Check sheet for the modelled part. Datum: model origin and axes. Units: mm. Face numbers are marked on the shaded views. A direction names the side the tool comes from. Round coordinates to 2 decimals unless told otherwise and drop trailing zeros. Order: outer loops, then holes, each group sorted by start corner. A loop starts at its lowest first (then second) coordinate and runs counter-clockwise, first axis right, second up.
Q1. Cross-section at A-A on z = 4. Record the cut outline in (x, y) (3 decimals), then the cut area to 4 significant figures.
Q2. Scan lines: probe 1 along X at (y, z) = (-0.5, 7); probe 2 along Y at (x, z) = (-26, 11.5); probe 3 along Y at (x, z) = (10.5, 3.5). Record each from-to range of solid material in increasing order.
Q3. Depth check by flat-ended pin: P1, Ø2, axis at y = -5.5, z = 6.5, coming from the +X side; P2, Ø13, axis at x = 0.5, z = 4, coming from the -Y side; P3, Ø2, axis at x = 34, z = 4.5, coming from the -Y side; P4, Ø10, axis at x = 38.5, y = -15, coming from the +Z side. Enter the tip coordinate at first touch or a pass-through.
Q4. Cross-section at C-C on z = 27. Record the cut outline in (x, y).
Q5. Set-up check for the marked faces 5 and 6: record each of +Z, -Z, +X, -X, +Y, -Y from which the full face is reachable in a straight line by a thin tool's end or side.
Q6. Mould release check, pull along X, two halves, no side actions. Record for the marked faces 1, 2, 3 and 4: +X half, -X half, draft (parallel to the pull), parting line (faces both ways), or undercut.
Q7. Cross-section at B-B on x = -20. Record the cut outline in (y, z).
Q8. Cross-section at D-D on y = -28.5. Record the cut outline in (x, z), then the cut area to 3 significant figures.
Autodesk Inventor part; units mm, degrees
ref_plane "YZ Plane" through (0, 0, 0) normal (1, 0, 0) x (0, 1, 0)
ref_plane "XZ Plane" through (0, 0, 0) normal (0, 1, 0) x (-1, 0, 0)
ref_plane "XY Plane" through (0, 0, 0) normal (0, 0, 1) x (1, 0, 0)
sketch "Sketch2" plane through (0, 0, 0) normal (0, 0, 1) x (1, 0, 0)
  line L0 (-32.475, -3.1) -> (-25.525, -3.1)
  line L1 (-25.525, -3.1) -> (-25.525, -7)
  line L2 (-25.525, -7) -> (-32.475, -7)
  line L3 (-32.475, -7) -> (-32.475, -3.1)
  line L4 (-31.2, 0) -> (-26.8, 0)
  line L5 (-26.8, 0) -> (-26.8, -3.1)
  line L6 (-26.8, -3.1) -> (-31.2, -3.1)
  line L7 (-31.2, -3.1) -> (-31.2, 0)
  line L8 (-35.5, 0) -> (0, 0)
  line L9 (0, 5) -> (-35.5, 5)
  line L10 (-35.5, 5) -> (-35.5, 0)
  line L11 (-29, 6.5254) -> (-29, -10.3092) construction
  line L12 (0, -40.9051) -> (0, 14.4305) construction
  line L13 (32.475, -3.1) -> (25.525, -3.1)
  line L14 (25.525, -3.1) -> (25.525, -7)
  line L15 (25.525, -7) -> (32.475, -7)
  line L16 (32.475, -7) -> (32.475, -3.1)
  line L17 (31.2, 0) -> (26.8, 0)
  line L18 (26.8, 0) -> (26.8, -3.1)
  line L19 (26.8, -3.1) -> (31.2, -3.1)
  line L20 (31.2, -3.1) -> (31.2, 0)
  line L21 (35.5, 0) -> (0, 0)
  line L22 (0, 5) -> (35.5, 5)
  line L23 (35.5, 5) -> (35.5, 0)
  line L24 (29, 6.5254) -> (29, -10.3092) construction
  line L25 (-85.0097, 0) -> (105.1151, 0) construction
  line L26 (35.5, 5) -> (77.9544, -30.0249)
  line L27 (77.9544, -30.0249) -> (75.5, -33)
  line L28 (75.5, -33) -> (35.5, 0)
  line L29 (-35.5, 5) -> (35.5, 5)
  line L30 (35.5, 5) -> (35.5, -7)
  line L31 (35.5, -7) -> (-35.5, -7)
  line L32 (-35.5, -7) -> (-35.5, 5)
  line L33 (-35.5, 5) -> (-57.849, -10.6443)
  line L34 (-57.849, -10.6443) -> (-55.5, -14)
  line L35 (-55.5, -14) -> (-35.5, 0)
  line L36 (-49.6567, -4.9097) -> (-47.3077, -8.2654)
  line L37 (-21.525, -7) -> (-21.525, -4)
  line L38 (-21.525, -4) -> (0, -4)
  line L39 (21.525, -7) -> (21.525, -4)
  line L40 (21.525, -4) -> (0, -4)
  line L41 (-35.5, -7) -> (-45.5, -7)
  line L42 (35.5, -7) -> (43.9848, -7)
  point P0 (-13.25, 5)
  point P1 (-18.25, 5)
  point P2 (29, -7)
  dimension "d1" = 4.4
  dimension "d2" = 6.95
  dimension "d3" = 3.9
  dimension "d4" = 5
  dimension "d5" = 58
  dimension "d6" = 7
  dimension "d7" = 13
  dimension "d28" = 38
  dimension "d29" = 40
  dimension "d30" = 20
  dimension "d31" = 19
  dimension "d32" = 10
  dimension "d37" = 4
  dimension "d38" = 3
extrude "Extrusion1" add sketch "Sketch2" along normal blind 12 contours L0 L1 L2 L3 | L7 L4 L5 L0 | L8 L10 L9 L22 L23 L21 L17 L4 | L35 L36 L33 L10 | L17 L20 L13 L18 | L14 L13 L16 L15 | L26 L27 L28 L23
extrude "Extrusion2" add sketch "Sketch2" along normal blind 40 contours L35 L34 L33 L36
extrude "Extrusion3" add sketch "Sketch2" against normal blind 3 contours L3 L31 L32 L8 L7 L0 | L0 L1 L2 L3 | L7 L4 L5 L0 | L5 L8 L21 L18 L13 L14 L31 L39 L40 L38 L37 L1 L0 | L8 L10 L9 L22 L23 L21 L17 L4 | L41 L35 L32 | L35 L36 L33 L10 | L35 L34 L33 L36 | L17 L20 L13 L18 | L14 L13 L16 L15 | L21 L30 L31 L16 L13 L20 | L26 L27 L28 L23 | L28 L42 L30
properties part number "UnitreeGO2_railmount"
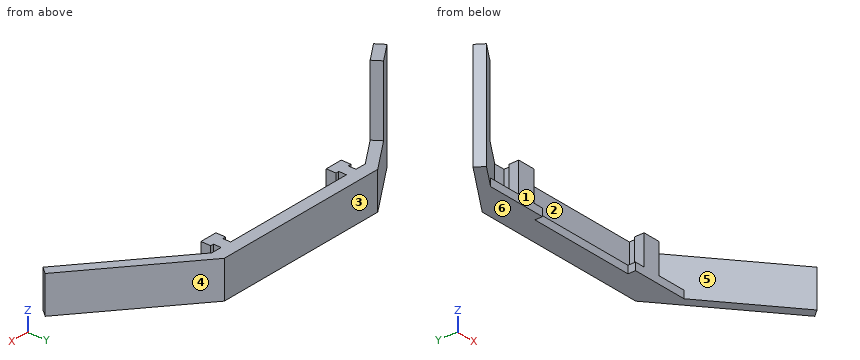
Results found:
1. outline: (-57.849, -10.644) - (-55.5, -14) - (-35.5, 0) - (-31.2, 0) - (-31.2, -3.1) - (-32.475, -3.1) - (-32.475, -7) - (-25.525, -7) - (-25.525, -3.1) - (-26.8, -3.1) - (-26.8, 0) - (26.8, 0) - (26.8, -3.1) - (25.525, -3.1) - (25.525, -7) - (32.475, -7) - (32.475, -3.1) - (31.2, -3.1) - (31.2, 0) - (35.5, 0) - (75.5, -33) - (77.954, -30.025) - (35.5, 5) - (-35.5, 5) - close
1. area: 748.5 mm2
2. probe 1: x = -43.36 to -36.21, -31.2 to -26.8, 26.8 to 31.2, 36.11 to 42.17
2. probe 2: y = -7 to -3.1, 0 to 5
2. probe 3: y = 0 to 5
3. P1: stops at x = 49.44
3. P2: stops at y = -4
3. P3: stops at y = 0
3. P4: passes through
4. outline: (-57.85, -10.64) - (-55.5, -14) - (-47.31, -8.27) - (-49.66, -4.91) - close
5. face 5: +Z, -Y
5. face 6: -Z, +X, -X, +Y, -Y
6. face 1: undercut
6. face 2: undercut
6. face 3: draft
6. face 4: +X half
7. outline: (-4, -3) - (5, -3) - (5, 12) - (0, 12) - (0, 0) - (-4, 0) - close
8. outline: (70.05, -3) - (76.11, -3) - (76.11, 12) - (70.05, 12) - close
8. area: 90.9 mm2
